```python
from build123d import *

# Parameters (mm, degrees)
BOSS_EXTRUDE1_DEPTH  = 3.175
M5_CLEARANCE_HOLE1_D = 5.5


with BuildPart() as part:
    # Sketch1 → Boss-Extrude1 (new body)
    with BuildSketch(Plane(origin=(0, 0, 0), x_dir=(1, 0, 0), z_dir=(0, 1, 0))):
        Polygon((0, 0), (73.025, 0), (73.025, 45.336003408), (0, 3.175), align=None)
    extrude(amount=BOSS_EXTRUDE1_DEPTH)

    # M5 Clearance Hole1 (through all)
    with Locations(Plane(origin=(0, 3.175, 0), x_dir=(1, 0, 0), z_dir=(0, 1, 0))):
        with Locations((19.05, 6.35), (66.675, 6.35)):
            Hole(M5_CLEARANCE_HOLE1_D / 2)


solid = part.part
```
The listing builds one solid part. Answer for the finished solid, in the listing's coordinates (mm). Coordinates: 2 decimals unless noted, no trailing zeros. Write each loop counter-clockwise with the first axis right and the second up, starting at its lowest first coordinate (ties: lowest second). Pieces come first, ordered by that corner, then holes.
Q1. The mould has two halves that part along Z. Classify faces 1 (the flat face through (36, 2, 0)), 2 (the cylindrical face through (17.57, 1.57, -8.67)), 3 (the flat face through (73.025, 2, -22)): released by +Z, released by -Z, zero draft, split by the parting line, or undercut.
Returned:
face 1: released by +Z
face 2: undercut
face 3: zero draft
Q2. Section B-B, the plane z = -7.5 is taken. Write down the section's boundary in (x, y) (3 decimals).
Returned:
outline: (7.491, 0) - (16.552, 0) - (16.552, 3.175) - (7.491, 3.175) - close; (21.548, 0) - (64.177, 0) - (64.177, 3.175) - (21.548, 3.175) - close; (69.173, 0) - (73.025, 0) - (73.025, 3.175) - (69.173, 3.175) - close
Q3. Find the intervals of material crossed by line 1 along Z through (x, y) = (19.05, 0.9); line 2 along X through (y, z) = (0.15, -39) (3 decimals); line 3 along X through (y, z) = (2.1, -38.5) (3 decimals), in increasing order.
Returned:
line 1: z = -14.17 to -9.1, -3.6 to 0
line 2: x = 62.051 to 73.025
line 3: x = 61.185 to 73.025
Q4. Section D-D, the plane x = 58.5 is taken. Write down the section's boundary in (y, z) (3 decimals), then the cut area to 3 significant figures.
Returned:
outline: (0, -36.95) - (3.175, -36.95) - (3.175, 0) - (0, 0) - close
area: 117 mm2
Q5. Section A-A, the plane x = 20.5 is taken. Write down the section's boundary in (y, z) (3 decimals), then the cut area to 3 significant figures.
Returned:
outline: (0, -15.011) - (3.175, -15.011) - (3.175, -8.687) - (0, -8.687) - close; (0, -4.013) - (3.175, -4.013) - (3.175, 0) - (0, 0) - close
area: 32.8 mm2
Q6. Given P1, Ø1, axis at y = 0.5, z = -19.5, coming from the -X side, flat-ended and moving along its own axis, determine where the tip first touches the part or whether it passes through.
Returned:
P1: stops at x = 27.41
Q7. Section C-C, the plane y = 1.55 is taken. Write down the section's boundary in (x, z) (3 decimals), then the cut area to 3 significant figures.
Returned:
outline: (0, -3.175) - (73.025, -45.336) - (73.025, 0) - (0, 0) - close; hole circle Ø5.5 at (19.05, -6.35); hole circle Ø5.5 at (66.675, -6.35)
area: 1,720 mm2
